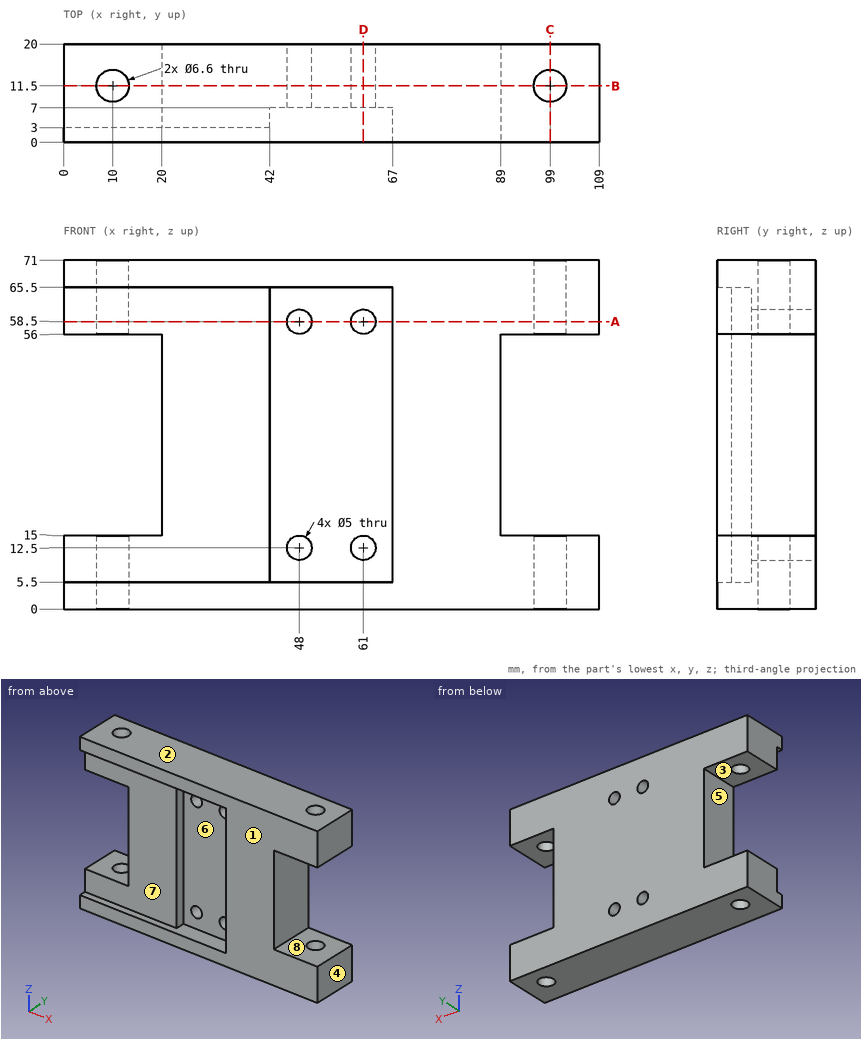
Study the drawing (mm; zero at the part's minimum x, y, z) and answer. A direction names the side the tool comes from. Round coordinates to 2 decimals unless told otherwise and drop trailing zeros. Loops run counter-clockwise (first coordinate to the right, second up) from the corner with the lowest first, then second, coordinate; pieces in that order, holes last.
Q1. Find the intervals of material crossed by line 1 (Z direction, x = 48, y = 14); line 2 (Z direction, x = 62.5, y = 18); line 3 (X direction, y = 4.25, z = 42.5), in increasing order.
Q2. Which of the six approach directions +Z, -Z, +X, -X, +Y, -Y give full straight-line access (tool end or side, diameter ignored) to the marked faces 4, 5, 6, 7 and 8?
Q3. Section B-B, the plane y = 11.5 is taken. Count the separate pieces of the cut face and the enclosed holes in it, then the cut area to 3 significant figures.
Q4. For a pull along Z with two mould halves and no side action, classify the marked faces 1, 2 and 3 as released by +Z, released by -Z, zero draft, split by the parting line, or undercut.
Q5. Section C-C, the plane x = 99 is taken. Determine the outline of the cut face in (y, z).
Q6. Section D-D, the plane x = 61 is taken. Determine the outline of the cut face in (y, z), then the cut area to 3 significant figures.
Q7. Section A-A, the plane z = 58.5 is taken. Determine the outline of the cut face in (x, y).
Q8. Given pin 1 Ø4 at (x, z) = (56, 18.5) entering from -Y; pin 2 Ø2 at (y, z) = (5, 49) entering from -X, each flat-ended and moving along its own axis, determine where each tip first touches the part or whether it passes through.
Completed:
1. line 1: z = 0 to 10, 15 to 56, 61 to 71
1. line 2: z = 0 to 10.5, 14.5 to 56.5, 60.5 to 71
1. line 3: x = 20 to 42, 67 to 89
2. face 4: +Z, -Z, +X, +Y, -Y
2. face 5: -X, +Y, -Y
2. face 6: -Y
2. face 7: -X, -Y
2. face 8: +X, +Y, -Y
3. separate pieces: 5
3. enclosed holes: 4
3. area: 5,620 mm2
4. face 1: zero draft
4. face 2: released by +Z
4. face 3: undercut
5. outline: (0, 0) - (8.2, 0) - (8.2, 15) - (0, 15) - close; (0, 56) - (8.2, 56) - (8.2, 71) - (0, 71) - close; (14.8, 0) - (20, 0) - (20, 15) - (14.8, 15) - close; (14.8, 56) - (20, 56) - (20, 71) - (14.8, 71) - close
6. outline: (0, 0) - (20, 0) - (20, 10) - (7, 10) - (7, 5.5) - (0, 5.5) - close; (0, 65.5) - (7, 65.5) - (7, 61) - (20, 61) - (20, 71) - (0, 71) - close; (7, 15) - (20, 15) - (20, 56) - (7, 56) - close
6. area: 870 mm2
7. outline: (0, 3) - (42, 3) - (42, 7) - (45.5, 7) - (45.5, 20) - (0, 20) - close; (50.5, 7) - (58.5, 7) - (58.5, 20) - (50.5, 20) - close; (63.5, 7) - (67, 7) - (67, 0) - (109, 0) - (109, 20) - (63.5, 20) - close; hole circle Ø6.6 at (10, 11.5); hole circle Ø6.6 at (99, 11.5)
8. pin 1: stops at y = 7
8. pin 2: stops at x = 20
